Check sheet for the modelled part. Datum: model origin and axes. Units: mm. A direction names the side the tool comes from. Round coordinates to 2 decimals unless told otherwise and drop trailing zeros. Write each loop counter-clockwise with the first axis right and the second up, starting at its lowest first coordinate (ties: lowest second). Pieces come first, ordered by that corner, then holes.
Item 1: Material ranges on line 1 (Y direction, x = 34.5, z = 1.3); line 2 (X direction, y = 55, z = 2.55); line 3 (Y direction, x = 29, z = 0.8), recorded low to high.
Item 2: Cross-section at A-A on x = 20.5. Enter the section's corners in (y, z), plus the area to 3 significant figures.
Item 3: Go/stop test with flat-tipped pins: pin 1 Ø1.8 at (y, z) = (107.5, 2) entering from +X; pin 2 Ø1.8 at (x, z) = (23, 2.5) entering from -Y; pin 3 Ø3 at (x, z) = (42, 2.5) entering from +Y. Record where each tip stops, or that it passes through.
Item 4: Cross-section at D-D on x = -65. Enter the section's corners in (y, z).
Item 5: Release check for a two-part mould opening along X. For faces 1 (the flat face through (29, -55, 3)), 2 (the cylindrical face through (25.577, -3.828, 2.958)), 3 (the flat face through (-15.5, -65, 3)), 4 (the flat face through (-64.4, 105.1, 3)) record: +X half, -X half, draft (parallel to the pull), parting line (faces both ways), or undercut.
Item 6: Cross-section at B-B on z = 2.5. Enter the section's corners in (x, y).
Item 7: Cross-section at C-C on y = -5. Enter the section's corners in (x, z), plus the area to 3 significant figures.
Item 8: Tool access check on faces 5 (the flat face through (28.87, -95.28, 2.96)), 6 (the flat face through (29, 105, 3)), 7 (the flat face through (30, -75, 3)). Record the directions out of +Z, -Z, +X, -X, +Y, -Y that give a thin tool (end or side, any length) a straight path to the whole face; none if there is none.
Autodesk Fusion 360 part; units mm, degrees
sketch "スケッチ1" plane through (0, 0, 0) normal (0, 0, 1) x (1, 0, 0)
  line L0 (-15.5, 115) -> (-74.5, 115)
  line L1 (-74.5, 115) -> (-74.5, -115)
  line L2 (-74.5, -115) -> (-15.5, -115)
  line L3 (74.5, -55) -> (74.5, 105)
  line L4 (68.0217, 105) -> (-74.5, -115) construction
  line L5 (-74.5, 115) -> (54.38, -83.9422) construction
  line L6 (-15.5, 115) -> (-15.5, 105)
  line L7 (-15.5, 105) -> (74.5, 105)
  line L8 (-74.5, -115) -> (-15.5, -115) construction
  line L9 (-15.5, -115) -> (74.5, -75)
  line L10 (74.5, -75) -> (-15.5, -75)
  line L11 (-15.5, -75) -> (-15.5, -55)
  line L12 (-15.5, -55) -> (74.5, -55)
  dimension "d2" = 230
  dimension "d5" = 59
  dimension "d7" = 90
  dimension "d8" = 20
extrude "押し出し1" add sketch "スケッチ1" along normal blind 6
chamfer "面取り1" distance 20 angle 45 2 edges at (-74.5, -115, 3) (-74.5, 115, 3)
sketch "スケッチ2" plane through (0, 0, 6) normal (0, 0, 1) x (-1, 0, 0)
  line L0 (54.5, -115) -> (74.5, -95)
  line L1 (74.5, -95) -> (74.5, 95)
  line L2 (74.5, 95) -> (54.5, 115)
  line L3 (54.5, 115) -> (15.5, 115)
  line L4 (15.5, 115) -> (-74.5, 75)
  line L5 (-74.5, 75) -> (15.5, 75)
  line L6 (15.5, 75) -> (15.5, 55)
  line L7 (15.5, 55) -> (-74.5, 55)
  line L8 (-74.5, 55) -> (-74.5, -105)
  line L9 (-74.5, -105) -> (15.5, -105)
  line L10 (15.5, -105) -> (15.5, -115)
  line L11 (15.5, -115) -> (54.5, -115)
  line L12 (-74.5, -105) -> (-34.5, -105) construction
  line L13 (-34.5, -105) -> (-34.5, -55) construction
  line L14 (-34.5, -55) -> (-74.5, -55) construction
  line L15 (-74.5, -55) -> (-74.5, -105) construction
  line L16 (-34.5, -55) -> (-34.5, 5) construction
  point P0 (-34.5, -55)
  point P1 (-34.5, 5)
  dimension "d12" = 40
  dimension "d13" = 50
  dimension "d14" = 60
hole "穴1" at (34.5, 55, 6) at (34.5, -5, 6) direction (0, 0, -1) diameter 18 end through all
equation "d5 = 20 mm + 39 mm"
Response values:
1. line 1: y = -92.78 to -75, -55 to -14, 4 to 46, 64 to 105
1. line 2: x = -74.5 to 25.5, 43.5 to 74.5
1. line 3: y = -95.22 to -75, -55 to -12.12, 2.12 to 47.88, 62.12 to 105
2. outline: (-99, 0) - (-75, 0) - (-75, 6) - (-99, 6) - close; (-55, 0) - (105, 0) - (105, 6) - (-55, 6) - close
2. area: 1,100 mm2
3. pin 1: stops at x = -15.5
3. pin 2: stops at y = -98.29
3. pin 3: stops at y = 105
4. outline: (-104.5, 0) - (104.5, 0) - (104.5, 6) - (-104.5, 6) - close
5. face 1: draft
5. face 2: undercut
5. face 3: +X half
5. face 4: -X half
6. outline: (-74.5, -95) - (-54.5, -115) - (-15.5, -115) - (74.5, -75) - (-15.5, -75) - (-15.5, -55) - (74.5, -55) - (74.5, 105) - (-15.5, 105) - (-15.5, 115) - (-54.5, 115) - (-74.5, 95) - close; hole circle Ø18 at (34.5, -5); hole circle Ø18 at (34.5, 55)
7. outline: (-74.5, 0) - (25.5, 0) - (25.5, 6) - (-74.5, 6) - close; (43.5, 0) - (74.5, 0) - (74.5, 6) - (43.5, 6) - close
7. area: 786 mm2
8. face 5: +Z, -Z, +X, -Y
8. face 6: +Z, -Z, +X, +Y
8. face 7: +Z, -Z, +X
